The figure shows three views and two pictorial views of one solid part (mm, origin at its lowest corner). Answer the questions. Round coordinates to 2 decimals unless told otherwise and drop trailing zeros. Write each loop counter-clockwise with the first axis right and the second up, starting at its lowest first coordinate (ties: lowest second). Pieces come first, ordered by that corner, then holes.
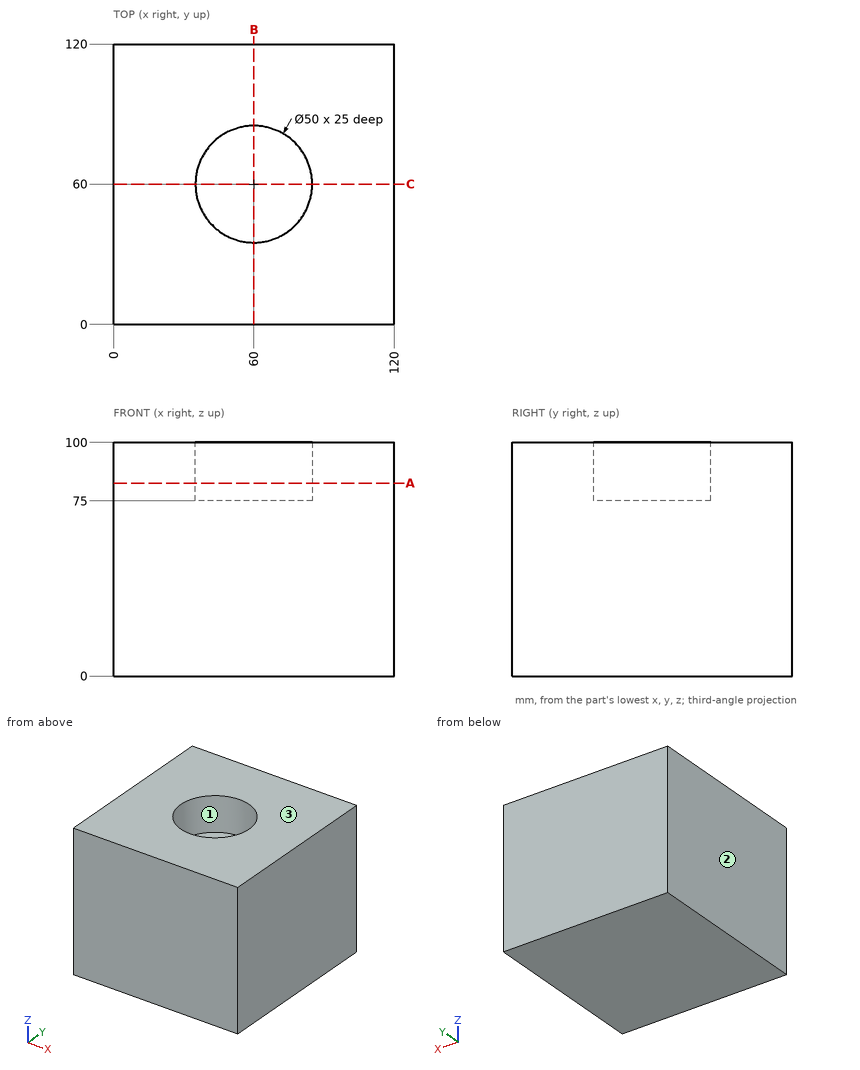
Q1. Determine the mould class of the marked faces 1, 2 and 3 for opening direction X: pulls with the +X half, pulls with the -X half, needs draft (parallel to the pull), parting line crosses it, or undercut.
Verdict:
face 1: undercut
face 2: pulls with the -X half
face 3: needs draft
Q2. Section A-A (z = 82.5) is taken. Determine the outline of the cut face in (x, y), then the cut area to 3 significant figures.
Verdict:
outline: (0, 0) - (120, 0) - (120, 120) - (0, 120) - close; hole circle Ø50 at (60, 60)
area: 12,400 mm2
Q3. Section B-B (x = 60) is taken. Determine the outline of the cut face in (y, z).
Verdict:
outline: (0, 0) - (120, 0) - (120, 100) - (85, 100) - (85, 75) - (35, 75) - (35, 100) - (0, 100) - close
Q4. Straight lines are drawn through the part: probe 1 along Y at (x, z) = (60, 88); probe 2 along X at (y, z) = (63.5, 82); probe 3 along Z at (x, y) = (57.5, 47.5). For each, find the intervals that lie inside material, in ascending order.
Verdict:
probe 1: y = 0 to 35, 85 to 120
probe 2: x = 0 to 35.25, 84.75 to 120
probe 3: z = 0 to 75
